Autodesk Fusion 360 part; units mm, degrees
sketch "Boceto1" plane through (0, 0, 0) normal (0, 0, 1) x (1, 0, 0)
  circle A0 centre (0, 0) radius 2.5
  line L0 (9.5, 6.0622) -> (0.5, 11.2583)
  line L1 (-0.5, 11.2583) -> (-9.5, 6.0622)
  line L2 (-10, 5.1962) -> (-10, -5.1962)
  line L3 (-9.5, -6.0622) -> (-0.5, -11.2583)
  line L4 (0.5, -11.2583) -> (9.5, -6.0622)
  line L5 (10, -5.1962) -> (10, 5.1962)
  line L6 (-2, 1.5) -> (2, 1.5)
  line L7 (-2, -1.5) -> (2, -1.5)
  arc A1 (-9.5, 6.0622) -> (-10, 5.1962) centre (-9, 5.1962) ccw
  arc A2 (0.5, 11.2583) -> (-0.5, 11.2583) centre (0, 10.3923) ccw
  arc A3 (10, 5.1962) -> (9.5, 6.0622) centre (9, 5.1962) ccw
  arc A4 (9.5, -6.0622) -> (10, -5.1962) centre (9, -5.1962) ccw
  arc A5 (-0.5, -11.2583) -> (0.5, -11.2583) centre (0, -10.3923) ccw
  arc A6 (-10, -5.1962) -> (-9.5, -6.0622) centre (-9, -5.1962) ccw
  dimension "d1" = 3
  dimension "d2" = 1.5
  dimension "d3" = 5
  dimension "d4" = 20
  dimension "d11" = 1
  dimension "d12" = 10
  dimension "d13" = 10
  dimension "d14" = 10
extrude "Extruir1" add sketch "Boceto1" along normal blind 20 contours A0 L6 L7
extrude "Extruir2" add sketch "Boceto1" against normal blind 10 contours A0 L6 L7 | A0 L6 | A0 L7 | L0 L1 L2 L3 L4 L5 A1 A2 A3 A4 A5 A6
fillet "Empalme1" radius 3 4 edges at (2.5, 0, 0) (0, -1.5, 0) (0, 1.5, 0) (-2.5, 0, 0)
equation "d2 = d1 / 2"
equation "d12 = d4 / 2"
For this review, take the finished solid that the model builds, in its own axes (mm). A direction names the side the tool comes from. Round coordinates to 2 decimals unless told otherwise and drop trailing zeros. Write each loop counter-clockwise with the first axis right and the second up, starting at its lowest first coordinate (ties: lowest second). Pieces come first, ordered by that corner, then holes. Notation, with made-up numbers: M -13.5,37 L 35.5,37 A30 cw 35.5,66 Z; hole C 41.5,15 d5. An arc over 180 degrees is marked long. One line per item, written item: value. Start each with the question number.
(1) We need section A-A (z = -8). Give the boundary of the cut face in (x, y), and give its area (3 significant figures).
(2) Wall thickness on line 1 (Z direction, x = 6, y = -1.75); line 2 (Y direction, x = 1.75, z = 11.5); line 3 (Y direction, x = 1.75, z = 2): over which ranges is each line inside the solid? List them lowest first.
(3) We need section B-B (x = -1.25). Give the boundary of the cut face in (y, z).
(4) We need section D-D (z = 14.25). Give the boundary of the cut face in (x, y), and give its area (3 significant figures).
(5) Machinability: for faces 1 (the flat face through (0, 1.5, 11)), 2 (the flat face through (0, 0, 20)), 3 (the flat face through (0, -5, 0)), 4 (the cylindrical face through (-2.5, 0, 11.4)), 5 (the flat face through (0, -1.5, 11)), which of the approach directions +Z, -Z, +X, -X, +Y, -Y give a long, thin tool a straight path to every point of the face, cutting with its end or side? Answer none if there is none.
(6) Insertion check: pin 1 (2 mm diameter, centred on x = -0.5, z = 9.5, fed in from +Y); pin 2 (10 mm diameter, centred on x = -0.5, z = 1, fed in from +Y); pin 3 (8 mm diameter, centred on x = 2.5, z = 16.5, fed in from -Y); pin 4 (4 mm diameter, centred on x = -3, y = 6.5, fed in from +Z). Each pin has a flat end and moves straight along its axis. Give the tip position at first contact, or say it passes through.
(7) We need section C-C (y = -7.5). Give the boundary of the cut face in (x, z).
Result:
1. outline: M -10,-5.2 A1 ccw -9.5,-6.06 L -0.5,-11.26 A1 ccw 0.5,-11.26 L 9.5,-6.06 A1 ccw 10,-5.2 L 10,5.2 A1 ccw 9.5,6.06 L 0.5,11.26 A1 ccw -0.5,11.26 L -9.5,6.06 A1 ccw -10,5.2 Z
1. area: 346 mm²
2. line 1: -10 to 0
2. line 2: -1.5 to 1.5
2. line 3: -1.67 to 1.67
3. outline: M -10.83,-10 L 10.83,-10 L 10.83,0 L 4.5,0 A3 cw 1.5,3 L 1.5,20 L -1.5,20 L -1.5,3 A3 cw -4.5,0 L -10.83,0 Z
4. outline: M -2,-1.5 L 2,-1.5 A2.5 ccw 2,1.5 L -2,1.5 A2.5 ccw Z
4. area: 14.0 mm²
5. face 1: +Z, +X, -X, +Y
5. face 2: +Z, +X, -X, +Y, -Y
5. face 3: +Z
5. face 4: +Z, -X
5. face 5: +Z, +X, -X, -Y
6. pin 1: y = 1.5
6. pin 2: y = 11.39
6. pin 3: y = -1.5
6. pin 4: z = 0
7. outline: M -7.01,-10 L 7.01,-10 L 7.01,0 L -7.01,0 Z
